from build123d import *

# Parameters (mm, degrees)
F1_DEPTH = 1041.4
F3_DEPTH = 127.001


# Not quite as in the source:
# - a feature names something its author has since deleted; it is built from what else it names


with BuildPart() as f1:
    # F0 (on Front) → F1 (new body)
    with BuildSketch(Plane.XZ):
        with BuildLine():
            ThreePointArc((0, 19.05), (5.5796158184, 5.5796158184), (19.05, 0))
            Line((19.05, 0), (107.95, 0))
            ThreePointArc((107.95, 0), (121.4203841816, 5.5796158184), (127, 19.05))
            Line((127, 19.05), (127, 107.95))
            ThreePointArc((127, 107.95), (121.4203841816, 121.4203841816), (107.95, 127))
            Line((107.95, 127), (19.05, 127))
            ThreePointArc((19.05, 127), (5.5796158184, 121.4203841816), (0, 107.95))
            Line((0, 107.95), (0, 19.05))
        make_face()
        with BuildLine():
            ThreePointArc((19.05, 9.525), (12.3148079092, 12.3148079092), (9.525, 19.05))
            Line((9.525, 19.05), (9.525, 107.95))
            ThreePointArc((9.525, 107.95), (12.3148079092, 114.6851920908), (19.05, 117.475))
            Line((19.05, 117.475), (107.95, 117.475))
            ThreePointArc((107.95, 117.475), (114.6851920908, 114.6851920908), (117.475, 107.95))
            Line((117.475, 107.95), (117.475, 19.05))
            ThreePointArc((117.475, 19.05), (114.6851920908, 12.3148079092), (107.95, 9.525))
            Line((107.95, 9.525), (19.05, 9.525))
        make_face(mode=Mode.SUBTRACT)
    extrude(amount=F1_DEPTH)

    # F2 (on Right) → F3 (cut, through all)
    with BuildSketch(Plane.YZ):
        Polygon((-1041.4, 19.05), (-1041.4, 0), (-968.0765158129, 127), (-1041.4, 127), (-1041.4, 107.95), align=None)
        Polygon((-73.3234841871, 127), (0, 0), (0, 19.05), (0, 107.95), (0, 127), align=None)
    extrude(amount=F3_DEPTH, mode=Mode.SUBTRACT)


solid = f1.part
Geometry: final body of the model. Coordinates: model frame, mm. A direction names the side the tool comes from. Give positions to 0.01 mm unless a question says otherwise; leave off trailing zeros. Loops run counter-clockwise (first coordinate to the right, second up) from the corner with the lowest first, then second, coordinate; pieces in that order, holes last. Notation, with made-up numbers: M -25.75,-16 L -8.75,-16 A23 cw -8.75,1 Z; hole C 33,-3 d11. An arc over 180 degrees is marked long. Put each result on its own line as item: value. Start each with the question number.
1) Ray query, line 1 along X through (y, z) = (-54, 81.5) (3 decimals); line 2 along X through (y, z) = (-882, 17). Return the intervals inside material, ascending.
2) Cut plane A-A (x = 49). Output: boundary loops of the cut face in (y, z) (3 decimals), then the cut area to 3 significant figures.
3) Contact query for a flat-ended pin moving along its axis: pin 1 (8 mm diameter, centred on y = -919.5, z = 41.5, fed in from -X). Output: stop coordinate, or through.
4) Pull-direction query (Z, two-part tool) for faces 3 (the flat face through (127, -514, 63)), 4 (the flat face through (117.475, -514, 64)), 5 (the flat face through (119.055, -37.175, 64.389)), 6 (the flat face through (63, -514, 117.475)); classes: pulls with the +Z half, pulls with the -Z half, needs draft (parallel to the pull), parting line crosses it, or undercut.
5) Cut plane B-B (z = 46). Output: boundary loops of the cut face in (x, y) (3 decimals), then the cut area to 3 significant figures.
6) Cut plane C-C (y = -708). Output: boundary loops of the cut face in (x, z) (3 decimals).
7) Access query for faces 1 (the flat face through (64, -513, 9.525)), 2 (the flat face through (119.06, -1005.25, 62.61)). Directions: +Z, -Z, +X, -X, +Y, -Y. A direction counts if a zero-diameter tool reaches every point of the face in a straight line with its end or side. Return the directions, or none.
Verdict:
1. line 1: 0 to 9.525, 117.475 to 127
1. line 2: 0.11 to 9.75, 117.25 to 126.89
2. outline: M -1041.4,0 L 0,0 L -5.499,9.525 L -1035.901,9.525 Z; M -973.576,117.475 L -67.824,117.475 L -73.323,127 L -968.077,127 Z
2. area: 18,400 mm2
3. pin 1: x = 0
4. face 3: needs draft
4. face 4: undercut
4. face 5: pulls with the +Z half
4. face 6: undercut
5. outline: M 0,-1014.842 L 9.525,-1014.842 L 9.525,-26.558 L 0,-26.558 Z; M 117.475,-1014.842 L 127,-1014.842 L 127,-26.558 L 117.475,-26.558 Z
5. area: 18,800 mm2
6. outline: M 0,19.05 A19.05 ccw 19.05,0 L 107.95,0 A19.05 ccw 127,19.05 L 127,107.95 A19.05 ccw 107.95,127 L 19.05,127 A19.05 ccw 0,107.95 Z; hole M 9.525,19.05 A9.525 ccw 19.05,9.525 L 107.95,9.525 A9.525 ccw 117.475,19.05 L 117.475,107.95 A9.525 ccw 107.95,117.475 L 19.05,117.475 A9.525 ccw 9.525,107.95 Z
7. face 1: +Y, -Y
7. face 2: +Z, +X, -X, -Y
